The model under review builds one solid part; all positions refer to its coordinate system, in mm. Round coordinates to 2 decimals unless told otherwise and drop trailing zeros. Order: outer loops, then holes, each group sorted by start corner. A loop starts at its lowest first (then second) coordinate and runs counter-clockwise, first axis right, second up.
```python
from build123d import *

# Parameters (mm, degrees)
F0_W     = 50
F0_H     = 100
F0_R     = 2.6
F0_R_2   = 2.1
F1_DEPTH = 3
F2_R     = 15
F3_R     = 2


with BuildPart() as f1:
    # F0 (on Top) → F1 (new body)
    with BuildSketch(Plane.XY):
        with Locations((-4.5, 0)):
            Rectangle(F0_W, F0_H)
        with Locations((-18.5, -30)):
            Circle(F0_R, mode=Mode.SUBTRACT)
        with Locations((-18.5, -10)):
            Circle(F0_R, mode=Mode.SUBTRACT)
        with Locations((0, -42.5)):
            Circle(F0_R_2, mode=Mode.SUBTRACT)
        with Locations((12.5, -14)):
            Circle(F0_R_2, mode=Mode.SUBTRACT)
        with Locations((-18.5, 10)):
            Circle(F0_R, mode=Mode.SUBTRACT)
        with Locations((-18.5, 30)):
            Circle(F0_R, mode=Mode.SUBTRACT)
        Circle(F0_R_2, mode=Mode.SUBTRACT)
        with Locations((12.5, 14)):
            Circle(F0_R_2, mode=Mode.SUBTRACT)
        with Locations((0, 42.5)):
            Circle(F0_R_2, mode=Mode.SUBTRACT)
    extrude(amount=F1_DEPTH)

    # F2
    f2_edges = [f1.edges().sort_by_distance(p)[0] for p in [
        (-29.5, -50, 1.5),
        (20.5, -50, 1.5),
        (20.5, 50, 1.5),
        (-29.5, 50, 1.5),
    ]]
    fillet(f2_edges, radius=F2_R)

    # F3
    f3_edges = [f1.edges().sort_by_distance(p)[0] for p in [
        (-4.5, 50, 3),
    ]]
    fillet(f3_edges, radius=F3_R)


solid = f1.part
```
(1) Consider section C-C (y = 11). Write out the cut boundary in (x, z), and give its area (3 significant figures).
Data:
outline: (-29.5, 0) - (-20.9, 0) - (-20.9, 3) - (-27.5, 3) arc R2 ccw to (-29.5, 1) - close; (-16.1, 0) - (20.5, 0) - (20.5, 1) arc R2 ccw to (18.5, 3) - (-16.1, 3) - close
area: 134 mm2
(2) Consider section D-D (x = 12.5). State how many separate pieces and enclosed holes the cut face has, and give its area (3 significant figures).
Data:
separate pieces: 3
enclosed holes: 0
area: 262 mm2
(3) Insertion check: pin 1 (3 mm diameter, centred on x = -18.5, y = -30, fed in from +Z). The pin has a flat end and moves straight along its axis. Give the tip position at first contact, or say it passes through.
Data:
pin 1: passes through
(4) Consider section A-A (y = -30). Write out the cut boundary in (x, z), and give its area (3 significant figures).
Data:
outline: (-29.5, 0) - (-21.1, 0) - (-21.1, 3) - (-27.5, 3) arc R2 ccw to (-29.5, 1) - close; (-15.9, 0) - (20.5, 0) - (20.5, 1) arc R2 ccw to (18.5, 3) - (-15.9, 3) - close
area: 133 mm2
(5) Draft analysis for pull direction X (two halves, no side actions). For faces 1 (the cylindrical face through (19.9, -0.49, 2.43)), 2 (the flat face through (-5, 1, 0)), 3 (the cylindrical face through (-17.3, -12.307, 1.479)), state which applies: pulls with the +X half, pulls with the -X half, needs draft (parallel to the pull), parting line crosses it, or undercut.
Data:
face 1: pulls with the +X half
face 2: needs draft
face 3: undercut
(6) To check wall thickness, follow probe 1 along Y at (x, z) = (-18.5, 1.9); probe 2 along Y at (x, z) = (13.5, 0.95); probe 3 along Y at (x, z) = (-18.5, 1.25). State the ranges of each line that lie inside material, in increasing order.
Data:
probe 1: y = -49.23 to -32.6, -27.4 to -12.6, -7.4 to 7.4, 12.6 to 27.4, 32.6 to 49.23
probe 2: y = -47.69 to -15.85, -12.15 to 12.15, 15.85 to 47.69
probe 3: y = -49.44 to -32.6, -27.4 to -12.6, -7.4 to 7.4, 12.6 to 27.4, 32.6 to 49.44
(7) Consider section B-B (x = 0). Write out the cut boundary in (y, z).
Data:
outline: (-50, 0) - (-44.6, 0) - (-44.6, 3) - (-48, 3) arc R2 ccw to (-50, 1) - close; (-40.4, 0) - (-2.1, 0) - (-2.1, 3) - (-40.4, 3) - close; (2.1, 0) - (40.4, 0) - (40.4, 3) - (2.1, 3) - close; (44.6, 0) - (50, 0) - (50, 1) arc R2 ccw to (48, 3) - (44.6, 3) - close
